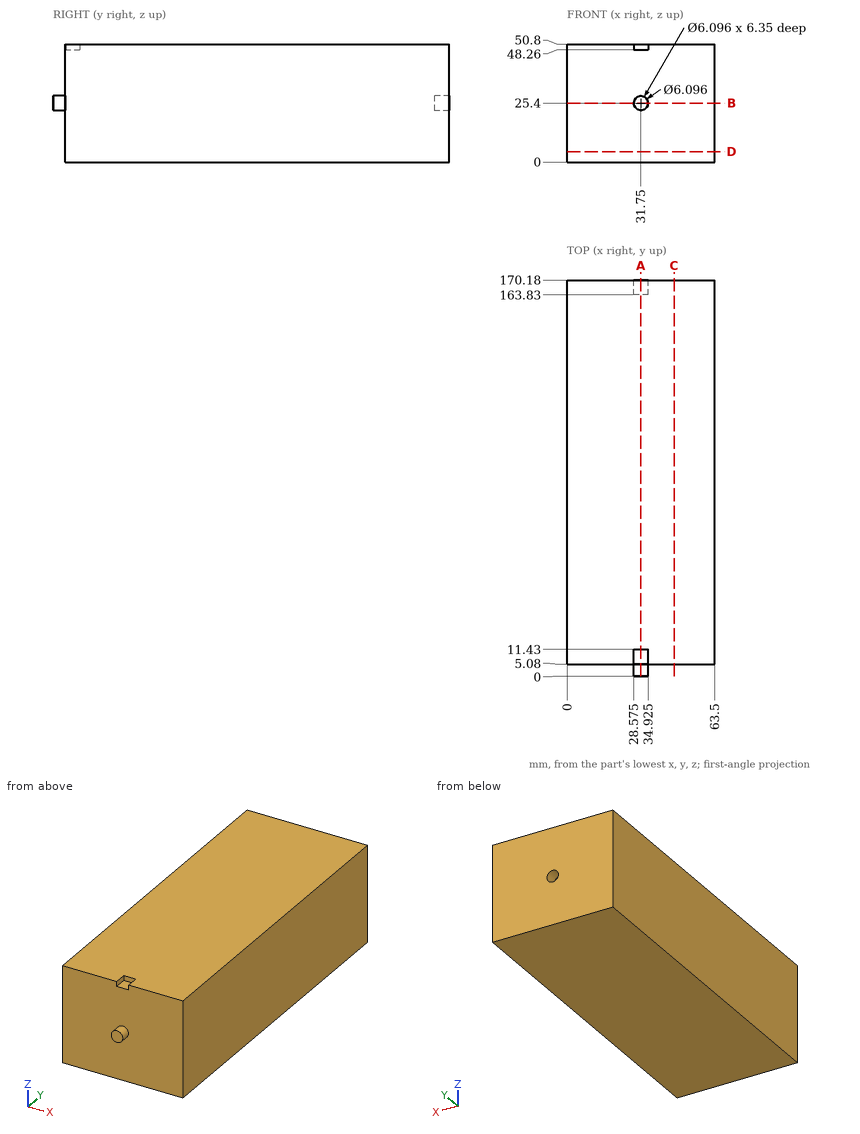
Part print with two shaded views. Sizes in mm from the minimum x, y, z corner. Round coordinates to 2 decimals unless told otherwise and drop trailing zeros. Write each loop counter-clockwise with the first axis right and the second up, starting at its lowest first coordinate (ties: lowest second). Pieces come first, ordered by that corner, then holes. Notation, with made-up numbers: M 28,-40 L 40,-40 A30 cw 40,-4 Z; hole C -36.5,-24.5 d2. An arc over 180 degrees is marked long. Put each result on its own line as item: value. Start each with the question number.
1) Pin check, flat tips, straight feed: pin 1 Ø3 at (x, z) = (7, 13.5) entering from -Y; pin 2 Ø2 at (x, z) = (31, 49.5) entering from -Y; pin 3 Ø3 at (x, z) = (32, 25) entering from +Y. Stop position of each tip, or through.
2) Saw through at D-D, the plane z = 4.5. Write the cut outline in (x, y).
3) Saw through at A-A, the plane x = 31.75. Write the cut outline in (y, z).
4) Saw through at B-B, the plane z = 25.4. Write the cut outline in (x, y), and give its area (3 significant figures).
5) Drill centre lines: probe 1 along X at (y, z) = (167, 25); probe 2 along Y at (x, z) = (35, 32.5); probe 3 along Z at (x, y) = (31, 167). Where is each one in solid material? Low to high. Write a range as [from, to].
6) Saw through at C-C, the plane x = 46. Write the cut outline in (y, z).
Resolved:
1. pin 1: y = 5.08
1. pin 2: y = 11.43
1. pin 3: y = 163.83
2. outline: M 0,5.08 L 63.5,5.08 L 63.5,170.18 L 0,170.18 Z
3. outline: M 0,22.35 L 5.08,22.35 L 5.08,0 L 170.18,0 L 170.18,22.35 L 163.83,22.35 L 163.83,28.45 L 170.18,28.45 L 170.18,50.8 L 11.43,50.8 L 11.43,48.26 L 5.08,48.26 L 5.08,28.45 L 0,28.45 Z
4. outline: M 0,5.08 L 28.7,5.08 L 28.7,0 L 34.8,0 L 34.8,5.08 L 63.5,5.08 L 63.5,170.18 L 34.8,170.18 L 34.8,163.83 L 28.7,163.83 L 28.7,170.18 L 0,170.18 Z
4. area: 10,500 mm²
5. probe 1: [0, 28.73], [34.77, 63.5]
5. probe 2: [5.08, 170.18]
5. probe 3: [0, 22.45], [28.35, 50.8]
6. outline: M 5.08,0 L 170.18,0 L 170.18,50.8 L 5.08,50.8 Z
